Here's the drawing with two shaded views (mm, measured from the low corner). I have some questions. Coordinates: 2 decimals unless noted, no trailing zeros. Order: outer loops, then holes, each group sorted by start corner. A loop starts at its lowest first (then second) coordinate and runs counter-clockwise, first axis right, second up. Notation, with made-up numbers: (17.25, -37.75) -> (46.25, -37.75) arc R12 ccw to (46.25, -26.75) -> close; hole circle Ø11 at (61.5, -23). An arc over 180 degrees is marked (long way). Answer as a JSON object with one key per item and string values. Group by question number.
(1) I want a section at B-B, the plane x = 348.5. List the corners of the cut face in (y, z) for me, plus the area to 3 significant figures.
(2) I need wall thicknesses on line 1 (Y direction, x = 59, z = 1.85); line 2 (Y direction, x = 68, z = 1.4); line 3 (X direction, y = 96, z = 2.85). Which ranges of each line are inside material? Lowest first, please.
(3) I want a section at A-A, the plane z = 0.65. List the corners of the cut face in (x, y) for me.
(4) For pin 1 (0.9 mm diameter, centred on x = 39, z = 1.5, fed in from +Y); pin 2 (0.9 mm diameter, centred on x = 20, z = 1, fed in from -Y); pin 3 (0.9 mm diameter, centred on x = 386, z = 1.5, fed in from -Y), each with a flat end and sliding along its axis, tell me the tip position at first contact or that it passes through.
(5) I want a section at C-C, the plane y = 109.5. List the corners of the cut face in (x, z) for me.
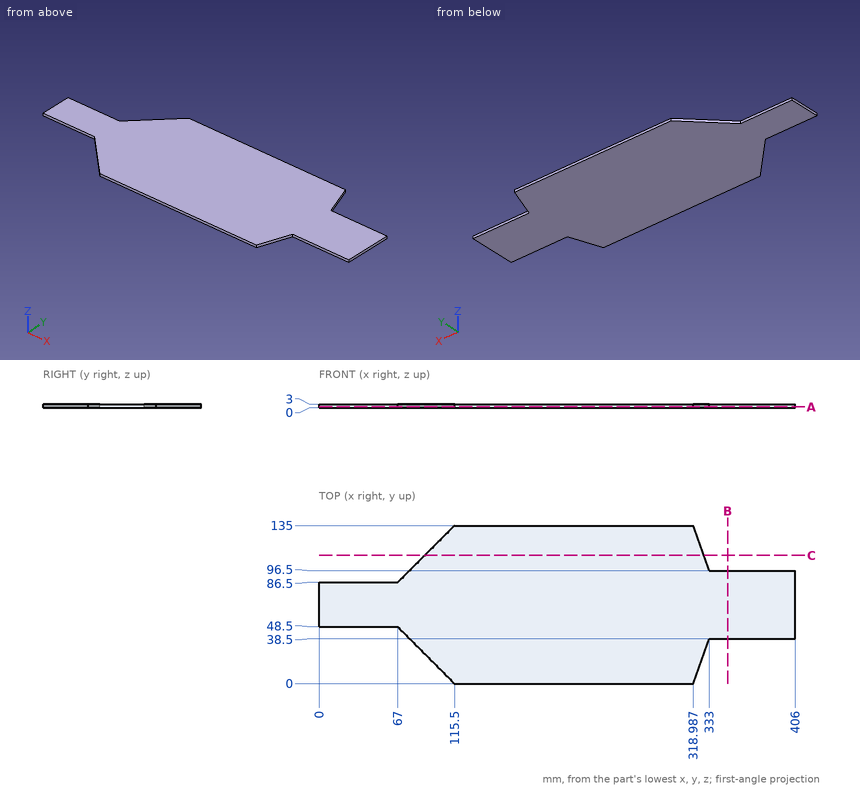
Computed values:
{
 "1": {"outline": "(38.5, 0) -> (96.5, 0) -> (96.5, 3) -> (38.5, 3) -> close", "area": "174 mm2"},
 "2": {"line 1": "y = 48.5 to 86.5", "line 2": "y = 47.5 to 87.5", "line 3": "x = 76.5 to 406"},
 "3": {"outline": "(0, 48.5) -> (67, 48.5) -> (115.5, 0) -> (318.99, 0) -> (333, 38.5) -> (406, 38.5) -> (406, 96.5) -> (333, 96.5) -> (318.99, 135) -> (115.5, 135) -> (67, 86.5) -> (0, 86.5) -> close"},
 "4": {"pin 1": "stops at y = 86.5", "pin 2": "stops at y = 48.5", "pin 3": "stops at y = 38.5"},
 "5": {"outline": "(90, 0) -> (328.27, 0) -> (328.27, 3) -> (90, 3) -> close"}
}
